Input: part model. Units: mm. Frame: model coordinates. Face numbers are marked on the shaded views. A direction names the side the tool comes from. Coordinates: 2 decimals unless noted, no trailing zeros. Write each loop counter-clockwise with the first axis right and the second up, starting at its lowest first coordinate (ties: lowest second). Pieces come first, ordered by that corner, then holes.
1) Draft query along X for the marked faces 1, 2 and 3. Return one class per face: pulls with the +X half, pulls with the -X half, needs draft (parallel to the pull), parting line crosses it, or undercut.
2) Section query C-C (z = -16.5). Output: boundary loops of the cut face in (x, y), then the cut area to 3 significant figures.
3) Set-up query: the marked faces 4, 5, 6 and 7. Return all of +Z, -Z, +X, -X, +Y, -Y with unobstructed straight access to the full face (end or side cutting, diameter ignored); none if empty.
4) Section query B-B (x = 20.33). Output: boundary loops of the cut face in (y, z), then the cut area to 3 significant figures.
5) Section query D-D (y = 7.63). Output: boundary loops of the cut face in (x, z), then the cut area to 3 significant figures.
6) Line query: L1, parallel to Z at x = 4, y = 3; L2, parallel to X at y = -4.7, z = -12.35; L3, parallel to Y at x = 6.35, z = -21.05. Output: solid intervals per line, ascending.
7) Section query A-A (y = 11.75). Output: boundary loops of the cut face in (x, z), then the cut area to 3 significant figures.
8) Pin query (flat end, axial travel): pin 1 Ø4 at (y, z) = (2.5, -15.5) entering from +X; pin 2 Ø1 at (y, z) = (14, -3.5) entering from -X; pin 3 Ø3 at (x, z) = (-1.5, -10) entering from +Y. Return the tip coordinate at first contact, or that it passes through.
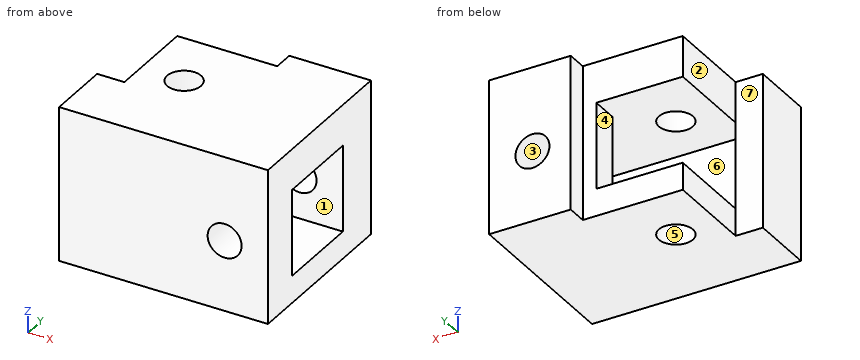
from build123d import *

# Parameters (mm, degrees)
SKETCH_1_W          = 26.7
SKETCH_1_H          = 22.7
EXTRUDE_1_DEPTH     = 6
SKETCH_1_3_W        = 26.7
SKETCH_1_3_H        = 6
SKETCH_1_3_H_2      = 4
EXTRUDE_2_DEPTH     = 12.7
SKETCH_2_R          = 2.5
CUT_EXTRUDE_1_DEPTH = 38.275595233
EXTRUDE_3_DEPTH     = 4
SKETCH_4_R          = 2.5
CUT_EXTRUDE_2_DEPTH = 42.754879954
SKETCH_6_W          = 22.7
SKETCH_6_H          = 9.5
EXTRUDE_4_DEPTH     = 4
EXTRUDE_START       = 3
SKETCH_7_W          = 12
SKETCH_7_H          = 22.7
SKETCH_7_R          = 2.5
EXTRUDE_5_DEPTH     = 3


with BuildPart() as part:
    # Sketch 1 → Extrude 1 (new body)
    with BuildSketch(Plane(origin=(0, 0, 0), x_dir=(1, 0, 0), z_dir=(0, 1, 0))):
        with Locations((13.35, 11.35)):
            Rectangle(SKETCH_1_W, SKETCH_1_H)
    extrude(amount=-EXTRUDE_1_DEPTH)

    # Sketch 1_3 → Extrude 2 (add)
    with BuildSketch(Plane(origin=(0, 0, 0), x_dir=(1, 0, 0), z_dir=(0, 1, 0))):
        with Locations((13.35, 3)):
            Rectangle(SKETCH_1_3_W, SKETCH_1_3_H)
        with Locations((13.35, 20.7)):
            Rectangle(SKETCH_1_3_W, SKETCH_1_3_H_2)
    extrude(amount=EXTRUDE_2_DEPTH)

    # Sketch 2 → Cut-Extrude 1 (cut, through all)
    with BuildSketch(Plane.XY):
        with Locations((6.35, 7.63)):
            Circle(SKETCH_2_R)
    extrude(amount=-CUT_EXTRUDE_1_DEPTH, mode=Mode.SUBTRACT)

    # Sketch 3 → Extrude 3 (add)
    with BuildSketch(Plane(origin=(0, 12.7, 0), x_dir=(1, 0, 0), z_dir=(0, 1, 0))):
        Polygon((0, 22.7), (0, 18.7), (12.7, 18.7), (12.7, 6), (0, 6), (0, 0), (26.7, 0), (26.7, 22.7), align=None)
    extrude(amount=EXTRUDE_3_DEPTH)

    # Sketch 4 → Cut-Extrude 2 (cut, through all)
    with BuildSketch(Plane(origin=(0, 16.7, 0), x_dir=(1, 0, 0), z_dir=(0, 1, 0))):
        with Locations(Location((20.33, 12.35, 0), (0, 0, 270))):
            Circle(SKETCH_4_R)
    extrude(amount=-CUT_EXTRUDE_2_DEPTH, mode=Mode.SUBTRACT)

    # Sketch 6 → Extrude 4 (add)
    with BuildSketch(Plane.ZY):
        with Locations((-11.35, -1.25)):
            Rectangle(SKETCH_6_W, SKETCH_6_H)
    extrude(amount=EXTRUDE_4_DEPTH)

    # Sketch 7 → Extrude 5 (add)
    with BuildSketch(Plane(origin=(0, 16.7, 0), x_dir=(1, 0, 0), z_dir=(0, 1, 0)).offset(EXTRUDE_START)):
        with Locations((20.7, 11.35)):
            Rectangle(SKETCH_7_W, SKETCH_7_H)
        with Locations(Location((20.33, 12.35, 0), (0, 0, 270))):
            Circle(SKETCH_7_R, mode=Mode.SUBTRACT)
    extrude(amount=-EXTRUDE_5_DEPTH)


solid = part.part
Answer:
1. face 1: needs draft
1. face 2: pulls with the -X half
1. face 3: undercut
2. outline: (-4, -6) - (26.7, -6) - (26.7, 0) - (0, 0) - (0, 3.5) - (-4, 3.5) - close; (12.7, 12.7) - (26.7, 12.7) - (26.7, 19.7) - (14.7, 19.7) - (14.7, 16.7) - (12.7, 16.7) - close
2. area: 290 mm2
3. face 4: -X, +Y
3. face 5: +Z, -Z
3. face 6: +X
3. face 7: +Z, -Z, -X, +Y
4. outline: (-6, -22.7) - (19.7, -22.7) - (19.7, -14.85) - (12.7, -14.85) - (12.7, -18.7) - (0, -18.7) - (0, -14.85) - (-6, -14.85) - close; (-6, -9.85) - (0, -9.85) - (0, -6) - (12.7, -6) - (12.7, -9.85) - (19.7, -9.85) - (19.7, 0) - (-6, 0) - close
4. area: 357 mm2
5. outline: (0, -22.7) - (3.85, -22.7) - (3.85, -18.7) - (0, -18.7) - close; (0, -6) - (3.85, -6) - (3.85, 0) - (0, 0) - close; (8.85, -22.7) - (26.7, -22.7) - (26.7, -18.7) - (8.85, -18.7) - close; (8.85, -6) - (26.7, -6) - (26.7, 0) - (8.85, 0) - close
5. area: 217 mm2
6. L1: z = -22.7 to -18.7, -6 to 0
6. L2: x = -4 to 17.83, 22.83 to 26.7
6. L3: y = -6 to 5.13, 10.13 to 16.7
7. outline: (0, -22.7) - (26.7, -22.7) - (26.7, -18.7) - (0, -18.7) - close; (0, -6) - (26.7, -6) - (26.7, 0) - (0, 0) - close
7. area: 267 mm2
8. pin 1: stops at x = 0
8. pin 2: stops at x = 0
8. pin 3: stops at y = 3.5
